from build123d import *

# Parameters (mm, degrees)
SKETCH1_W           = 1460
SKETCH1_H           = 600
BOSS_EXTRUDE1_DEPTH = 40
FILLET1_R           = 10
CUT_EXTRUDE1_REACH  = 792.253
SKETCH2_W           = 304
SKETCH2_H           = 344


with BuildPart() as part:
    # Sketch1 → Boss-Extrude1 (new body)
    with BuildSketch(Plane(origin=(0, 0, 0), x_dir=(1, 0, 0), z_dir=(0, 1, 0))):
        Rectangle(SKETCH1_W, SKETCH1_H)
    extrude(amount=BOSS_EXTRUDE1_DEPTH)

    # Fillet1
    fillet1_edges = [part.edges().sort_by_distance(p)[0] for p in [
        (0, 40, 300),
    ]]
    fillet(fillet1_edges, radius=FILLET1_R)

    # Sketch2 → Cut-Extrude1 (cut, up to next)
    with BuildSketch(Plane(origin=(0, 40, 0), x_dir=(1, 0, 0), z_dir=(0, 1, 0)), mode=Mode.PRIVATE) as cut_extrude1_sk1:
        with Locations((-530, -58)):
            Rectangle(SKETCH2_W, SKETCH2_H)
    cut_extrude1_tool1 = extrude(cut_extrude1_sk1.sketch, amount=-CUT_EXTRUDE1_REACH, mode=Mode.PRIVATE) & part.part
    add(cut_extrude1_tool1.solids().sort_by_distance((-530, 40, 58))[0], mode=Mode.SUBTRACT)


solid = part.part
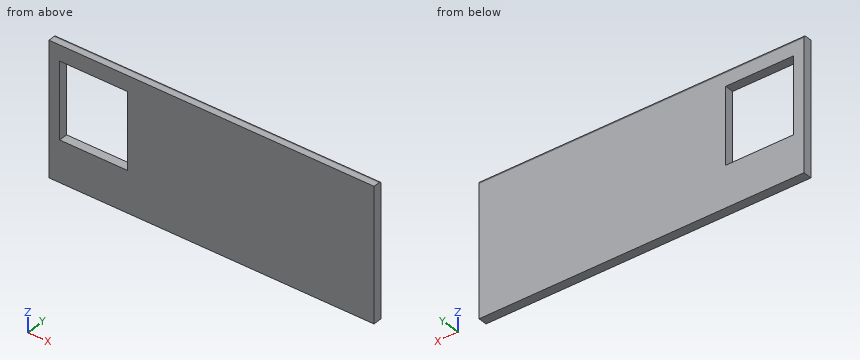
The model under review builds one solid part; all positions refer to its coordinate system, in mm. Give positions to 0.01 mm unless a question says otherwise; leave off trailing zeros. Order: outer loops, then holes, each group sorted by start corner. A loop starts at its lowest first (then second) coordinate and runs counter-clockwise, first axis right, second up. Notation, with made-up numbers: M -24.75,44.25 L 7.25,44.25 A14 cw 7.25,70.25 Z; hole C 44,-12.5 d6. An arc over 180 degrees is marked long. Answer in a Markdown table with one row per item. Add a question column.
1. Add section A-A on z = 25.5. State the section outline as (x, y) points.
2. Add section B-B on x = -533. State the section outline as (y, z) points, plus the area to 3 significant figures.
3. To check wall thickness, follow line 1 along Z through (x, y) = (-571.5, 10.5); line 2 along X through (y, z) = (36.5, 78.5); line 3 along Z through (x, y) = (383, 38). State the ranges of each line that lie inside material, in increasing order.
4. Add section C-C on y = 17. State the section outline as (x, z) points.
5. For pin 1 Ø1.5 at (x, y) = (283, 35.5) entering from +Z; pin 2 Ø1.5 at (x, y) = (-397, 34.5) entering from +Z, all flat-tipped, find the tip position at first contact; note any pin that passes through.
The answers:
| question | item | result |
|---|---|---|
| 1 | outline | M -730,0 L -682,0 L -682,40 L -730,40 Z; M -378,0 L 730,0 L 730,40 L -378,40 Z |
| 2 | outline | M 0,-300 L 40,-300 L 40,-114 L 0,-114 Z; M 0,230 L 40,230 L 40,290 A10 ccw 30,300 L 0,300 Z |
| 2 | area | 10,200 mm2 |
| 3 | line 1 | -300 to -114, 230 to 300 |
| 3 | line 2 | -730 to -682, -378 to 730 |
| 3 | line 3 | -300 to 296 |
| 4 | outline | M -730,-300 L 730,-300 L 730,300 L -730,300 Z; hole M -682,-114 L -378,-114 L -378,230 L -682,230 Z |
| 5 | pin 1 | z = 298.8 |
| 5 | pin 2 | z = 299.27 |
